from build123d import *

# Parameters (mm, degrees)
F0_R     = 38.1
F3_DEPTH = 127
F2_R     = 21.245809
F4_DEPTH = 127.001
F1_W     = 42.491618
F1_H     = 42.491618
F5_DEPTH = 25.4


with BuildPart() as f3:
    # F0 (on Front) → F3 (new body)
    with BuildSketch(Plane.XZ):
        Circle(F0_R)
    extrude(amount=-F3_DEPTH)

    # F2 (on Front) → F4 (cut, through all)
    with BuildSketch(Plane.XZ):
        Circle(F2_R)
    extrude(amount=-F4_DEPTH, mode=Mode.SUBTRACT)

    # F1 (on Front) → F5 (cut)
    with BuildSketch(Plane.XZ):
        Rectangle(F1_W, F1_H)
    extrude(amount=-F5_DEPTH, mode=Mode.SUBTRACT)


solid = f3.part
The listing builds one solid part. Answer for the finished solid, in the listing's coordinates (mm). A direction names the side the tool comes from. Give positions to 0.01 mm unless a question says otherwise; leave off trailing zeros. Write each loop counter-clockwise with the first axis right and the second up, starting at its lowest first coordinate (ties: lowest second). Pieces come first, ordered by that corner, then holes.
Item 1: Section A-A, the plane x = 8 is taken. Write down the section's boundary in (y, z), plus the area to 3 significant figures.
Item 2: Section D-D, the plane z = -25 is taken. Write down the section's boundary in (x, y), plus the area to 3 significant figures.
Item 3: Determine the mould class of faces 3 (the flat face through (-21.246, 13, 0)), 4 (the flat face through (16, 127, -16)), 5 (the cylindrical face through (-30.235, 62.611, -23.183)) for opening direction X: released by +X, released by -X, zero draft, split by the parting line, or undercut.
Item 4: Section C-C, the plane y = 54 is taken. Write down the section's boundary in (x, z), plus the area to 3 significant figures.
Item 5: Find the intervals of material crossed by line 1 along Z through (x, y) = (0, 61); line 2 along X through (y, z) = (19, -1.5); line 3 along X through (y, z) = (10, -19), in increasing order.
Item 6: Section B-B, the plane z = 11 is taken. Write down the section's boundary in (x, y).
Item 7: Flat-ended cylindrical pins translate along their axes: P1, Ø20.5, axis at y = 9.5, z = 3, coming from the +X side; P2, Ø1.5, axis at x = -28, y = 18, coming from the -Z side; P3, Ø1.5, axis at x = 30, y = 27.5, coming from the +Z side; P4, Ø4, axis at x = -6.5, y = 35, coming from the +Z side. Find the tip coordinate at first contact, or state that the pin passes through.
Item 8: Which of the six approach directions +Z, -Z, +X, -X, +Y, -Y give full straight-line access (tool end or side, diameter ignored) to faces 1 (the flat face through (0, 13, 21.246)), 2 (the flat face through (-1, 0, -25))?
Completed:
1. outline: (0, -37.25) - (127, -37.25) - (127, -19.68) - (25.4, -19.68) - (25.4, -21.25) - (0, -21.25) - close; (0, 21.25) - (25.4, 21.25) - (25.4, 19.68) - (127, 19.68) - (127, 37.25) - (0, 37.25) - close
1. area: 4,380 mm2
2. outline: (-28.75, 0) - (28.75, 0) - (28.75, 127) - (-28.75, 127) - close
2. area: 7,300 mm2
3. face 3: undercut
3. face 4: zero draft
3. face 5: split by the parting line
4. outline: circle Ø76.2 at (0, 0); hole circle Ø42.49 at (0, 0)
4. area: 3,140 mm2
5. line 1: z = -38.1 to -21.25, 21.25 to 38.1
5. line 2: x = -38.07 to -21.25, 21.25 to 38.07
5. line 3: x = -33.02 to -21.25, 21.25 to 33.02
6. outline: (-36.48, 0) - (-21.25, 0) - (-21.25, 25.4) - (-18.18, 25.4) - (-18.18, 127) - (-36.48, 127) - close; (18.18, 25.4) - (21.25, 25.4) - (21.25, 0) - (36.48, 0) - (36.48, 127) - (18.18, 127) - close
7. P1: stops at x = 38.1
7. P2: stops at z = -26.63
7. P3: stops at z = 24.41
7. P4: stops at z = 37.83
8. face 1: -Y
8. face 2: +Z, -Z, +X, -X, -Y
